Autodesk Inventor part; units mm, degrees
ref_plane "YZ Plane" through (0, 0, 0) normal (1, 0, 0) x (0, 1, 0)
ref_plane "XZ Plane" through (0, 0, 0) normal (0, 1, 0) x (-1, 0, 0)
ref_plane "XY Plane" through (0, 0, 0) normal (0, 0, 1) x (1, 0, 0)
sketch "草图1" plane through (0, 0, 0) normal (0, 0, 1) x (1, 0, 0)
  circle A0 centre (0, 0) radius 4
  dimension "d0" = 8
extrude "拉伸1" add sketch "草图1" along normal blind 1
sketch "草图2" plane through (0, 0, 1) normal (0, 0, 1) x (1, 0, 0)
  line L0 (1.7321, -3) -> (-1.7321, -3)
  line L1 (-1.7321, -3) -> (-3.4641, 0)
  line L2 (-3.4641, 0) -> (-1.7321, 3)
  line L3 (-1.7321, 3) -> (1.7321, 3)
  line L4 (1.7321, 3) -> (3.4641, 0)
  line L5 (3.4641, 0) -> (1.7321, -3)
  line L6 (0, 0) -> (0, 3)
  dimension "d3" = 6
extrude "拉伸2" add sketch "草图2" along normal blind 4
sketch "草图3" plane through (0, 0, 0) normal (0, 0, -1) x (-1, 0, 0)
  circle A0 centre (0, 0) radius 2.5
  dimension "d6" = 5
extrude "拉伸3" add sketch "草图3" along normal blind 14
thread "螺纹1"
chamfer "倒角1" distance 0.25 angle 45 1 edges at (2.5, 0, -14)
properties part number "分离水箱固定螺丝"
For this review, take the finished solid that the model builds, in its own axes (mm). A direction names the side the tool comes from. Round coordinates to 2 decimals unless told otherwise and drop trailing zeros. Write each loop counter-clockwise with the first axis right and the second up, starting at its lowest first coordinate (ties: lowest second). Pieces come first, ordered by that corner, then holes. Notation, with made-up numbers: (36.25, 13.25) - (50.25, 13.25) arc R17 cw to (50.25, 29.25) - close; hole circle Ø2 at (11.25, 67). An arc over 180 degrees is marked (long way). Use a Markdown table: item, result.
Q1. The part is to be moulded in two halves that separate along X. For faces 5 (the cylindrical face through (0.54, 2.44, -6.78)), 6 (the flat face through (-2.6, -1.5, 3)), 7 (the flat face through (2.6, 1.5, 3)), 8 (the flat face through (0, 0, 5)), say which applies: pulls with the +X half, pulls with the -X half, needs draft (parallel to the pull), parting line crosses it, or undercut.
Derived:
| item | result |
|---|---|
| face 5 | parting line crosses it |
| face 6 | pulls with the -X half |
| face 7 | pulls with the +X half |
| face 8 | needs draft |
Q2. We need section A-A (x = 0). Give the boundary of the cut face in (y, z), plus the area to 3 significant figures.
Derived:
| item | result |
|---|---|
| outline | (-4, 0) - (-2.5, 0) - (-2.5, -13.75) - (-2.25, -14) - (2.25, -14) - (2.5, -13.75) - (2.5, 0) - (4, 0) - (4, 1) - (3, 1) - (3, 5) - (-3, 5) - (-3, 1) - (-4, 1) - close |
| area | 102 mm2 |
Q3. We need section D-D (z = -4.75). Give the boundary of the cut face in (x, y).
Derived:
| item | result |
|---|---|
| outline | circle Ø5 at (0, 0) |
Q4. Clearance check with a flat-ended pin moving along its axis: pin 1 (1 mm diameter, centred on x = 0.5, z = 3.5, fed in from +Y). State where the tip first meets the part, or that it passes through.
Derived:
| item | result |
|---|---|
| pin 1 | stops at y = 3 |
Q5. We need section B-B (z = 1.75). Give the boundary of the cut face in (x, y), plus the area to 3 significant figures.
Derived:
| item | result |
|---|---|
| outline | (-3.46, 0) - (-1.73, -3) - (1.73, -3) - (3.46, 0) - (1.73, 3) - (-1.73, 3) - close |
| area | 31.2 mm2 |
Q6. Wall thickness on line 1 along Z through (x, y) = (2.5, 3); line 2 along Z through (x, y) = (2, -2.25); line 3 along X through (y, z) = (-0.25, -6.5): over which ranges is each line inside the solid? List them lowest first.
Derived:
| item | result |
|---|---|
| line 1 | z = 0 to 1 |
| line 2 | z = 0 to 5 |
| line 3 | x = -2.49 to 2.49 |
Q7. Machinability: for faces 1 (the flat face through (3, 2, 1)), 2 (the flat face through (0, -3, 3)), 3 (the flat face through (-2.6, 1.5, 3)), 4 (the flat face through (2.6, -1.5, 3)), which of the approach directions +Z, -Z, +X, -X, +Y, -Y give a long, thin tool a straight path to every point of the face, cutting with its end or side? Answer none if there is none.
Derived:
| item | result |
|---|---|
| face 1 | +Z |
| face 2 | +Z, +X, -X, -Y |
| face 3 | +Z, -X, +Y |
| face 4 | +Z, +X, -Y |
Q8. We need section C-C (y = 2.75). Give the boundary of the cut face in (x, z).
Derived:
| item | result |
|---|---|
| outline | (-2.9, 0) - (2.9, 0) - (2.9, 1) - (1.88, 1) - (1.88, 5) - (-1.88, 5) - (-1.88, 1) - (-2.9, 1) - close |
